```python
from build123d import *

# Parameters (mm, degrees)
SKETCH_1_W      = 9.6
SKETCH_1_H      = 9.6
EXTRUDE_1_DEPTH = 4.5
SKETCH_3_R      = 0.25
EXTRUDE_3_DEPTH = 4.5
SKETCH_4_R      = 1.15
EXTRUDE_4_DEPTH = 1.5


with BuildPart() as part:
    # 草图1 → 拉伸1 (new body)
    with BuildSketch(Plane(origin=(0, 0, 0), x_dir=(1, 0, 0), z_dir=(0, 1, 0))):
        Rectangle(SKETCH_1_W, SKETCH_1_H)
    extrude(amount=EXTRUDE_1_DEPTH)

    # 草图3 → 拉伸3 (add)
    with BuildSketch(Plane(origin=(0, 0, -4.8), x_dir=(-1, 0, 0), z_dir=(0, 0, -1))):
        with Locations(Location((0, 2.25, 0), (0, 0, 180))):
            Circle(SKETCH_3_R)
        with Locations(Location((2.595978382, 2.25, 0), (0, 0, 180))):
            Circle(SKETCH_3_R)
        with Locations(Location((-2.595978382, 2.25, 0), (0, 0, 180))):
            Circle(SKETCH_3_R)
    extrude(amount=EXTRUDE_3_DEPTH)

    # 草图4 → 拉伸4 (add)
    with BuildSketch(Plane.XY.offset(4.8)):
        with Locations(Location((-3.3, 3, 0), (0, 0, 180))):
            Circle(SKETCH_4_R)
    extrude(amount=EXTRUDE_4_DEPTH)


solid = part.part
```
Geometry check sheet. Reference: the model listing, model coordinates, mm. A direction names the side the tool comes from. Coordinates: 2 decimals unless noted, no trailing zeros. Loops run counter-clockwise (first coordinate to the right, second up) from the corner with the lowest first, then second, coordinate; pieces in that order, holes last.
Item 1: Sectioned sample at D-D, the plane y = 2.25. Record the boundary of the cut face in (x, z), then the cut area to 3 significant figures.
Item 2: Sectioned sample at B-B, the plane y = 3. Record the boundary of the cut face in (x, z).
Item 3: Sectioned sample at C-C, the plane z = -7. Record the boundary of the cut face in (x, y), then the cut area to 3 significant figures.
Item 4: Thickness scan on line 1 (Z direction, x = -1, y = 2.2); line 2 (Y direction, x = 0, z = -7.5); line 3 (Z direction, x = -3.25, y = 2). Record the ranges inside material, lowest first.
Item 5: Sectioned sample at A-A, the plane x = -3.3. Record the boundary of the cut face in (y, z).
Item 6: Go/stop test with a flat-tipped pin: pin 1 Ø1.3 at (x, y) = (1.5, 2) entering from -Z. Record where the tip stops, or that it passes through.
Item 7: Access from +Z, -Z, +X, -X, +Y, -Y to the whole of each face (thin tool, end or side, straight path). Record for faces 1 (the face through (4.8, 2, 0)), 2 (the face through (-4.362, 3.44, 5.54)).
Check result:
1. outline: (-4.8, -4.8) - (-2.85, -4.8) - (-2.85, -9.3) - (-2.35, -9.3) - (-2.35, -4.8) - (-0.25, -4.8) - (-0.25, -9.3) - (0.25, -9.3) - (0.25, -4.8) - (2.35, -4.8) - (2.35, -9.3) - (2.85, -9.3) - (2.85, -4.8) - (4.8, -4.8) - (4.8, 4.8) - (-2.43, 4.8) - (-2.43, 6.3) - (-4.17, 6.3) - (-4.17, 4.8) - (-4.8, 4.8) - close
1. area: 102 mm2
2. outline: (-4.8, -4.8) - (4.8, -4.8) - (4.8, 4.8) - (-2.15, 4.8) - (-2.15, 6.3) - (-4.45, 6.3) - (-4.45, 4.8) - (-4.8, 4.8) - close
3. outline: circle Ø0.5 at (-2.6, 2.25); circle Ø0.5 at (0, 2.25); circle Ø0.5 at (2.6, 2.25)
3. area: 0.589 mm2
4. line 1: z = -4.8 to 4.8
4. line 2: y = 2 to 2.5
4. line 3: z = -4.8 to 6.3
5. outline: (0, -4.8) - (4.5, -4.8) - (4.5, 4.8) - (4.15, 4.8) - (4.15, 6.3) - (1.85, 6.3) - (1.85, 4.8) - (0, 4.8) - close
6. pin 1: stops at z = -4.8
7. face 1: +Z, -Z, +X, +Y, -Y
7. face 2: +Z
